CAD build for the part. Positions are in the model's coordinates, mm. A direction names the side the tool comes from. Round coordinates to 2 decimals unless told otherwise and drop trailing zeros. Order: outer loops, then holes, each group sorted by start corner. A loop starts at its lowest first (then second) coordinate and runs counter-clockwise, first axis right, second up.
Autodesk Inventor part; units mm, degrees
ref_plane "YZ Plane" through (0, 0, 0) normal (1, 0, 0) x (0, 1, 0)
ref_plane "XZ Plane" through (0, 0, 0) normal (0, 1, 0) x (-1, 0, 0)
ref_plane "XY Plane" through (0, 0, 0) normal (0, 0, 1) x (1, 0, 0)
sketch "Sketch1" plane through (0, 0, 0) normal (0, 1, 0) x (-1, 0, 0)
  line L0 (16, 17.5) -> (-16, 17.5)
  line L1 (-16, 17.5) -> (-16, -17.5)
  line L2 (-16, -17.5) -> (16, -17.5)
  line L3 (16, -17.5) -> (16, 17.5)
  line L4 (16, 17.5) -> (-16, -17.5) construction
  line L5 (-16, 17.5) -> (16, -17.5) construction
  line L6 (0, -17.5) -> (0, -14.5) construction
  line L7 (0, -14.5) -> (3, -14.5) construction
  circle A0 centre (3, -14.5) radius 2
  circle A1 centre (-3, -14.5) radius 2
  point P0 (0, 0)
  dimension "d0" = 32
  dimension "d1" = 35
  dimension "d5" = 3
  dimension "d6" = 3
  dimension "d7" = 4
extrude "Extrusion1" add sketch "Sketch1" along normal blind 72 contours L3 L2 L1 L0 | A0 | A1
extrude "Extrusion2" add sketch "Sketch1" along normal blind 15 from surface at 72 contours A0 | A1
fillet "Fillet1" radius 3 12 edges at (16, 36, 17.5) (16, 36, -17.5) (-16, 36, 17.5) (-16, 36, -17.5) (16, 72, 0) (0, 72, 17.5) (0, 72, -17.5) (-16, 72, 0) (16, 0, 0) (0, 0, 17.5) (-16, 0, 0) (0, 0, -17.5)
properties part number "SLS Quantum 1300mAh 4S1P 14,8V 65C"
1. Drill centre lines: line 1 (Y direction, x = -5, z = -11); line 2 (Z direction, x = 9, y = 70.5); line 3 (X direction, y = 70, z = -5). Where is each one in solid material? Low to high.
2. Mould opens along X. For faces 1 (the face through (3.26, 79.008, -16.483)), 2 (the face through (15.1, 0.86, 0.2)), 3 (the face through (0, 36, -17.5)), 4 (the face through (-15.14, 35.54, -16.6)) say: released by +X, released by -X, zero draft, split by the parting line, or undercut.
3. Cut at C-C, the plane x = -10. Write the cut outline in (y, z).
4. Pin check, flat tips, straight feed: P1, Ø12, axis at x = 5, z = 3, coming from the +Y side; P2, Ø6, axis at y = 73.5, z = 12.5, coming from the +X side. Stop position of each tip, or through.
5. Tool access for faces 5 (the face through (0.18, 71.1, -16.64)), 6 (the face through (0, 0, 0)): list every direction of +Z, -Z, +X, -X, +Y, -Y with a clear straight run to the whole face (end or side of a thin tool).
6. Cut at B-B, the plane z = 0.5. Write the cut outline in (x, y).
7. Cut at A-A, the plane x = 3. Write the cut outline in (y, z), and give its area (3 significant figures).
Outcome:
1. line 1: y = 0 to 72
1. line 2: z = -17.1 to 17.1
1. line 3: x = -15.83 to 15.83
2. face 1: undercut
2. face 2: released by +X
2. face 3: zero draft
2. face 4: released by -X
3. outline: (0, -14.5) arc R3 ccw to (3, -17.5) - (69, -17.5) arc R3 ccw to (72, -14.5) - (72, 14.5) arc R3 ccw to (69, 17.5) - (3, 17.5) arc R3 ccw to (0, 14.5) - close
4. P1: stops at y = 72
4. P2: stops at x = 15.6
5. face 5: -Z, +Y
5. face 6: +Z, -Z, +X, -X, -Y
6. outline: (-16, 3) arc R3 ccw to (-13, 0) - (13, 0) arc R3 ccw to (16, 3) - (16, 69) arc R3 ccw to (13, 72) - (-13, 72) arc R3 ccw to (-16, 69) - close
7. outline: (0, -14.5) arc R3 ccw to (3, -17.5) - (69, -17.5) arc R3 ccw to (71.24, -16.5) - (87, -16.5) - (87, -12.5) - (72, -12.5) - (72, 14.5) arc R3 ccw to (69, 17.5) - (3, 17.5) arc R3 ccw to (0, 14.5) - close
7. area: 2,570 mm2
